from build123d import *

# Parameters (mm, degrees)
F0_W      = 38.1
F0_H      = 38.1
F1_DEPTH  = 38.1
F6_DEPTH  = 38.1
F8_DEPTH  = 38.1
F9_W      = 25.270408
F9_H      = 7.62
F9_W_2    = 25.464796
F10_DEPTH = 38.1


with BuildPart() as f1:
    # F0 (on Front) → F1 (new body)
    with BuildSketch(Plane.XZ):
        with Locations((19.05, 19.05)):
            Rectangle(F0_W, F0_H)
    extrude(amount=F1_DEPTH)

    # F5 (on offset) → F6 (cut)
    with BuildSketch(Plane.YZ.offset(38.1)):
        Polygon((-31.75, 0), (-38.1, 38.1), (-38.1, 0), align=None)
        Polygon((-25.4, 0), (-12.7, 0), (-19.05, 16.622577), align=None)
        Polygon((-11.43, 16.622577), (-6.35, 38.1), (-31.75, 38.1), (-26.67, 16.622577), (-21.59, 30.142272), (-16.51, 30.142272), align=None)
        Polygon((-6.35, 0), (0, 0), (0, 38.1), align=None)
    extrude(amount=-F6_DEPTH, mode=Mode.SUBTRACT)

    # F7 (on offset) → F8 (cut)
    with BuildSketch(Plane.XZ.offset(38.1)):
        Polygon((0, 38.1), (0, 0), (6.35, 38.1), align=None)
        Polygon((25.4, 38.1), (12.7, 38.1), (19.05, 22.225), align=None)
        Polygon((11.43, 22.225), (6.35, 0), (31.75, 0), (26.67, 22.225), (21.59, 9.525), (16.51, 9.525), align=None)
        Polygon((31.75, 38.1), (38.1, 0), (38.1, 38.1), align=None)
    extrude(amount=-F8_DEPTH, mode=Mode.SUBTRACT)

    # F9 (on offset) → F10 (cut)
    with BuildSketch(Plane.XY.offset(38.1)):
        with Locations((25.464796, -11.43)):
            Rectangle(F9_W, F9_H)
        with Locations((12.732398, -26.67)):
            Rectangle(F9_W_2, F9_H)
    extrude(amount=-F10_DEPTH, mode=Mode.SUBTRACT)


solid = f1.part
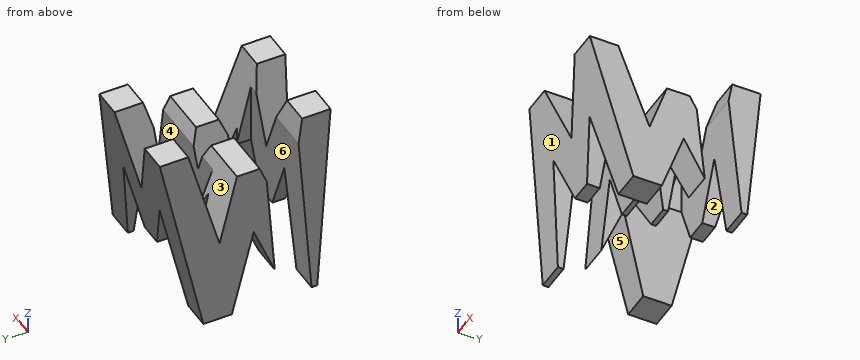
Can you work these out from the model? Positions are in its coordinate system, mm. Face numbers are marked on the shaded views. A direction names the side the tool comes from. Give positions to 0.01 mm unless a question says otherwise; leave off trailing zeros. Order: outer loops, then holes, each group sorted by start corner. A loop starts at its lowest first (then second) coordinate and runs counter-clockwise, first axis right, second up. Notation, with made-up numbers: M 61.25,55.5 L 112.25,55.5 A10 cw 112.25,64.5 Z; hole C 82.5,22.5 d2. An arc over 180 degrees is marked long. Use one line per item in the form item = value.
Item 1: If we section it at C-C, the plane y = -7: Write out the boundary of the cut face in (x, z) (3 decimals), and give its area (3 significant figures).
Values follow:
outline = M 0,0 L 6.35,0 L 11.43,22.225 L 16.51,9.525 L 21.59,9.525 L 26.67,22.225 L 31.75,0 L 38.1,0 L 32.208,35.352 L 24.301,35.352 L 19.05,22.225 L 13.799,35.352 L 5.892,35.352 Z
area = 747 mm^2
Item 2: For the marked faces 4, 5 and 6, which set-ups out of +Z, -Z, +X, -X, +Y, -Y let a thin tool reach every point of the face, with its end or its side?
Values follow:
face_4 = +Z, -Z, +X
face_5 = -Z, +X, -X
face_6 = +Z, -Z, -X
Item 3: If we section it at B-B, the plane x = 3.5: Write out the boundary of the cut face in (y, z), and give its area (3 significant figures).
Values follow:
outline = M -35.25,21 L -31.75,0 L -30.48,0 L -30.48,21 Z; M -22.86,6.65 L -19.05,16.62 L -12.7,0 L -6.35,0 L -2.85,21 L -10.39,21 L -11.43,16.62 L -13.07,21 L -22.86,21 Z
area = 344 mm^2
Item 4: If we section it at D-D, the plane x = 26: Write out the boundary of the cut face in (y, z) (3 decimals), and give its area (3 significant figures).
Values follow:
outline = M -38.1,38.1 L -35.175,20.55 L -27.599,20.55 L -31.75,38.1 Z; M -25.194,20.55 L -15.24,20.55 L -15.24,26.762 L -16.51,30.142 L -21.59,30.142 Z; M -7.62,20.55 L -2.925,20.55 L 0,38.1 L -6.35,38.1 L -7.62,32.731 Z
area = 303 mm^2
Item 5: If I drill on line 1 along Y through (x, z) = (6, 18.5); line 2 along Y through (x, z) = (27, 25); line 3 along X through (y, z) = (-33.5, 17.5), over which ranges is the centre line in solid material (lowest first)? Write a range as [from, to].
Values follow:
line_1 = [-34.83, -30.48], [-22.86, -12.14], [-10.99, -3.27]
line_2 = [-35.92, -28.65], [-23.52, -15.24], [-7.62, -2.18]
line_3 = [2.92, 10.35], [13.32, 24.78], [27.75, 35.18]
Item 6: Thinking about a two-plate mould opening in Y: for the marked faces 1, 2 and 3, which applies, pulls with the +Y half, pulls with the -Y half, needs draft (parallel to the pull), parting line crosses it, or undercut?
Values follow:
face_1 = pulls with the -Y half
face_2 = needs draft
face_3 = undercut
Item 7: Will these pins go through, and if not, where does the flat tip stop? pin 1 Ø4 at (x, z) = (9, 30) entering from +Y; pin 2 Ø20.5 at (x, z) = (14.5, 23) entering from +Y; pin 3 Ø6 at (x, z) = (17, 18) entering from -Y; pin 4 Ø1 at (y, z) = (-10, 28) entering from +X.
Values follow:
pin_1 = -1.02
pin_2 = -0.81
pin_3 = -35.25
pin_4 = through
Item 8: If we section it at A-A, the plane z = 8: Write out the boundary of the cut face in (x, y).
Values follow:
outline = M 1.33,-33.08 L 8.18,-33.08 L 8.18,-30.48 L 1.33,-30.48 Z; M 1.33,-22.86 L 8.18,-22.86 L 8.18,-22.34 L 1.33,-22.34 Z; M 1.33,-15.76 L 8.18,-15.76 L 8.18,-5.02 L 1.33,-5.02 Z; M 29.92,-33.08 L 36.77,-33.08 L 36.77,-22.34 L 29.92,-22.34 Z; M 29.92,-15.76 L 36.77,-15.76 L 36.77,-15.24 L 29.92,-15.24 Z; M 29.92,-7.62 L 36.77,-7.62 L 36.77,-5.02 L 29.92,-5.02 Z
